The listing builds one solid part. Answer for the finished solid, in the listing's coordinates (mm). Face numbers are marked on the shaded views. A direction names the side the tool comes from. Round coordinates to 2 decimals unless told otherwise and drop trailing zeros. Loops run counter-clockwise (first coordinate to the right, second up) from the corner with the lowest first, then second, coordinate; pieces in that order, holes last. Notation, with made-up numbers: (-36.75, 40.5) - (10.25, 40.5) arc R25 ccw to (10.25, 57.5) - close; hole circle Ø10 at (-27, 66). An arc over 180 degrees is marked (long way). Write item = value, one per line. Start each with the question number.
1) A tool of negligible diameter and unlimited length cuts with its end or side. For the marked faces 1, 2 and 3, from which of +Z, -Z, +X, -X, +Y, -Y can it reach the whole face along a straight path? Write none if from no direction.
2) Section B-B, the plane x = 0 is taken. Determine the outline of the cut face in (y, z), and give its area (3 significant figures).
3) Section A-A, the plane z = 0.5 is taken. Determine the outline of the cut face in (x, y), and give its area (3 significant figures).
4) Straight lines are drawn through the part: line 1 along Z through (x, y) = (0.1, 0); line 2 along Y through (x, z) = (-2.25, -0.9); line 3 along X through (y, z) = (8.5, -1.5). For each, find the intervals that lie inside material, in ascending order.
5) Section C-C, the plane y = -15 is taken. Determine the outline of the cut face in (x, z), and give its area (3 significant figures).
6) Given pin 1 Ø3 at (x, y) = (1, -9) entering from -Z; pin 2 Ø3 at (y, z) = (-5, -2) entering from +X, each flat-ended and moving along its own axis, determine where each tip first touches the part or whether it passes through.
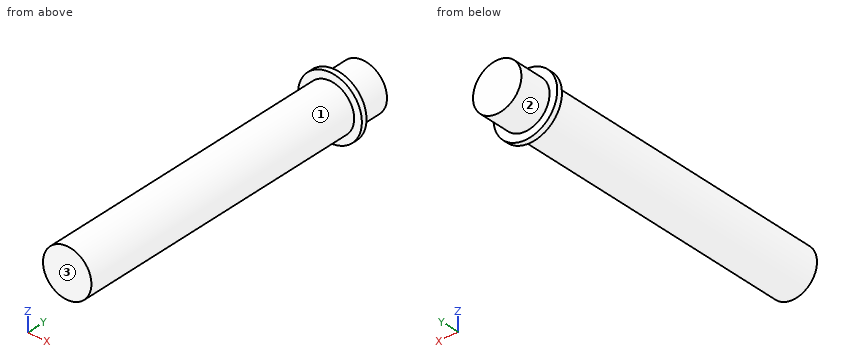
from build123d import *

# Parameters (mm, degrees)
BOSS_EXTRUDE1_DEPTH      = 10
BOSS_EXTRUDE1_DEPTH_BACK = 21.5
SKETCH1_R                = 2.2
SKETCH2_R                = 2.9
SKETCH2_R_2              = 2.2
BOSS_EXTRUDE2_DEPTH      = 0.5


with BuildPart() as part:
    # Sketch1 → Boss-Extrude1 (new, two sides: drawn at the far end of the back side and taken through both)
    with BuildSketch(Plane(origin=(0, 0, 0), x_dir=(1, 0, 0), z_dir=(0, 1, 0)).offset(-BOSS_EXTRUDE1_DEPTH_BACK)):
        with Locations(Location((0, 0, 0), (0, 0, 270))):
            Circle(SKETCH1_R)
    extrude(amount=BOSS_EXTRUDE1_DEPTH + BOSS_EXTRUDE1_DEPTH_BACK)

    # Sketch2 → Boss-Extrude2 (add)
    with BuildSketch(Plane(origin=(0, 7, 0), x_dir=(1, 0, 0), z_dir=(0, 1, 0))):
        with Locations(Location((0, 0, 0), (0, 0, 270))):
            Circle(SKETCH2_R)
        with Locations(Location((0, 0, 0), (0, 0, 270))):
            Circle(SKETCH2_R_2, mode=Mode.SUBTRACT)
    extrude(amount=-BOSS_EXTRUDE2_DEPTH)


solid = part.part
Geometry check:
q1.face_1 = -Y
q1.face_2 = +Y
q1.face_3 = +Z, -Z, +X, -X, -Y
q2.outline = (-21.5, -2.2) - (6.5, -2.2) - (6.5, -2.9) - (7, -2.9) - (7, -2.2) - (10, -2.2) - (10, 2.2) - (7, 2.2) - (7, 2.9) - (6.5, 2.9) - (6.5, 2.2) - (-21.5, 2.2) - close
q2.area = 139 mm2
q3.outline = (-2.86, 6.5) - (-2.14, 6.5) - (-2.14, -21.5) - (2.14, -21.5) - (2.14, 6.5) - (2.86, 6.5) - (2.86, 7) - (2.14, 7) - (2.14, 10) - (-2.14, 10) - (-2.14, 7) - (-2.86, 7) - close
q3.area = 136 mm2
q4.line_1 = -2.2 to 2.2
q4.line_2 = 6.5 to 7
q4.line_3 = -1.61 to 1.61
q5.outline = circle Ø4.4 at (0, 0)
q5.area = 15.2 mm2
q6.pin_1 = -2.2
q6.pin_2 = 2.14
